Input: part model. Units: mm. Frame: model coordinates. Face numbers are marked on the shaded views. A direction names the side the tool comes from. Coordinates: 2 decimals unless noted, no trailing zeros. Order: outer loops, then holes, each group sorted by start corner. A loop starts at its lowest first (then second) coordinate and runs counter-clockwise, first axis right, second up. Notation, with made-up numbers: (21, 81.25) - (79, 81.25) arc R25 cw to (79, 97.25) - close; hole circle Ø6 at (15.5, -36.5). An arc over 180 degrees is marked (long way). Use a Markdown table: item, result. Add a question column.
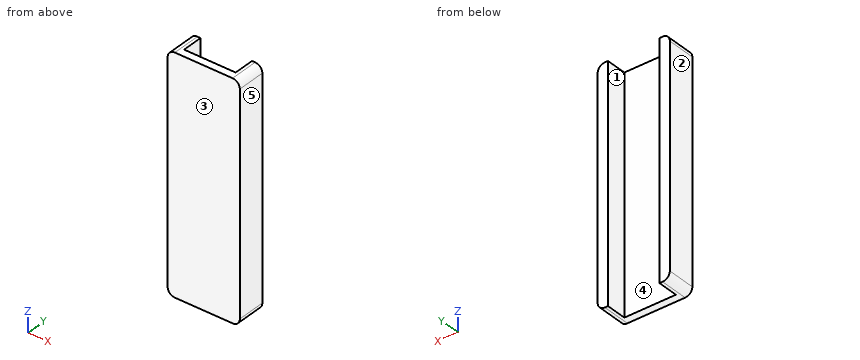
from build123d import *

# Parameters (mm, degrees)
SKETCH_1_W      = 14
SKETCH_1_H      = 45
EXTRUDE_1_DEPTH = 1.5
SKETCH_2_W      = 2
SKETCH_2_H      = 45
EXTRUDE_2_DEPTH = 4
FILLET_1_R      = 1.4


with BuildPart() as part:
    # 草图1 → 凸台-拉伸1 (new body)
    with BuildSketch(Plane(origin=(0, 0, 0), x_dir=(1, 0, 0), z_dir=(0, 1, 0))):
        with Locations((7, 22.5)):
            Rectangle(SKETCH_1_W, SKETCH_1_H)
    extrude(amount=EXTRUDE_1_DEPTH)

    # 草图2 → 凸台-拉伸2 (add)
    with BuildSketch(Plane(origin=(0, 1.5, 0), x_dir=(1, 0, 0), z_dir=(0, 1, 0))):
        with Locations((1, 22.5)):
            Rectangle(SKETCH_2_W, SKETCH_2_H)
        with Locations((13, 22.5)):
            Rectangle(SKETCH_2_W, SKETCH_2_H)
    extrude(amount=EXTRUDE_2_DEPTH)

    # 圆角1
    fillet_1_edges = [part.edges().sort_by_distance(p)[0] for p in [
        (0, 2.75, -45),
        (14, 2.75, -45),
        (14, 2.75, 0),
        (0, 2.75, 0),
    ]]
    fillet(fillet_1_edges, radius=FILLET_1_R)


solid = part.part
1) Cut plane A-A (y = 4.5). Return the cut outline in (x, z).
2) Contact query for flat-ended pins moving along their axis: P1, Ø8, axis at x = 3, z = -6.5, coming from the -Y side; P2, Ø1, axis at x = 11, z = -13, coming from the +Y side. Output: stop coordinate, or through.
3) Cut plane B-B (z = -5). Return the cut outline in (x, y), and give its area (3 significant figures).
4) Reachability of the marked faces 4 and 5 from +Z, -Z, +X, -X, +Y, -Y: full face, straight path, thin tool, end or side. Return the list, or none.
5) Cut plane C-C (x = 4). Return the cut outline in (y, z), and give its area (3 significant figures).
6) Material intervals for L1, parallel to X at y = 3.6, z = -16; L2, parallel to Y at x = 3.75, z = -6; L3, parallel to Z at x = 12.75, y = 3.4, sorted ascending.
7) Pull-direction query (X, two-part tool) for the marked faces 1, 2 and 3; classes: pulls with the +X half, pulls with the -X half, needs draft (parallel to the pull), parting line crosses it, or undercut.
Computed:
| question | item | result |
|---|---|---|
| 1 | outline | (0, -43.6) arc R1.4 ccw to (1.4, -45) - (2, -45) - (2, 0) - (1.4, 0) arc R1.4 ccw to (0, -1.4) - close; (12, -45) - (12.6, -45) arc R1.4 ccw to (14, -43.6) - (14, -1.4) arc R1.4 ccw to (12.6, 0) - (12, 0) - close |
| 2 | P1 | stops at y = 0 |
| 2 | P2 | stops at y = 1.5 |
| 3 | outline | (0, 0) - (14, 0) - (14, 5.5) - (12, 5.5) - (12, 1.5) - (2, 1.5) - (2, 5.5) - (0, 5.5) - close |
| 3 | area | 37.0 mm2 |
| 4 | face 4 | +Z, -Z, +Y |
| 4 | face 5 | +Z, -Z, +X, +Y, -Y |
| 5 | outline | (0, -45) - (1.5, -45) - (1.5, 0) - (0, 0) - close |
| 5 | area | 67.5 mm2 |
| 6 | L1 | x = 0 to 2, 12 to 14 |
| 6 | L2 | y = 0 to 1.5 |
| 6 | L3 | z = -44.99 to -0.01 |
| 7 | face 1 | undercut |
| 7 | face 2 | pulls with the -X half |
| 7 | face 3 | needs draft |
